Autodesk Inventor part; units mm, degrees
ref_plane "YZ Plane" through (0, 0, 0) normal (1, 0, 0) x (0, 1, 0)
ref_plane "XZ Plane" through (0, 0, 0) normal (0, 1, 0) x (-1, 0, 0)
ref_plane "XY Plane" through (0, 0, 0) normal (0, 0, 1) x (1, 0, 0)
sketch "Sketch1" plane through (0, 0, 0) normal (0, 0, 1) x (1, 0, 0)
  line L0 (0, 0) -> (71, 0)
  line L1 (71, 0) -> (71, 72.4)
  line L2 (71, 72.4) -> (0, 72.4)
  line L3 (0, 72.4) -> (0, 0)
  dimension "d0" = 71
  dimension "d1" = 72.4
extrude "Extrusion1" add sketch "Sketch1" along normal blind 10
sketch "Sketch2" plane through (0, 0, 10) normal (0, 0, 1) x (1, 0, 0)
  line L0 (71, 0) -> (71, 72.4)
  line L1 (71, 12.4) -> (81, 12.4)
  line L2 (81, 12.4) -> (81, 52.4)
  line L3 (81, 52.4) -> (71, 52.4)
  line L4 (71, 52.4) -> (71, 12.4)
  line L5 (71, 72.4) -> (0, 72.4)
  circle A0 centre (76, 32.4) radius 2.5
  line L6 (0, 0) -> (71, 0)
  point P0 (81, 32.4)
  point P1 (76, 52.4)
  dimension "d4" = 10
  dimension "d5" = 40
  dimension "d7" = 5
  dimension "d53" = 20
extrude "Extrusion2" add sketch "Sketch2" against normal blind 10
sketch "Sketch3" plane through (0, 0, 10) normal (0, 0, 1) x (1, 0, 0)
  line L0 (71, 52.4) -> (81, 52.4)
  line L1 (71, 12.4) -> (81, 12.4)
  line L2 (81, 52.4) -> (71, 52.4)
  line L3 (71, 52.4) -> (71, 12.4)
  line L4 (71, 12.4) -> (81, 12.4)
  line L5 (81, 12.4) -> (81, 52.4)
  point P0 (0, 0)
extrude "Extrusion3" cut sketch "Sketch3" against normal blind 5
sketch "Sketch10" plane through (0, 0, 0) normal (0, 0, -1) x (-1, 0, 0)
  line L0 (0, 72.4) -> (0, 0)
  line L1 (0, 12.4) -> (10, 12.4)
  line L2 (10, 12.4) -> (10, 52.4)
  line L3 (10, 52.4) -> (0, 52.4)
  line L4 (0, 52.4) -> (0, 12.4)
  circle A0 centre (5, 32.4) radius 2.5
  point P0 (-81, 12.4)
  point P1 (10, 32.4)
  point P2 (5, 12.4)
  dimension "d40" = 10
  dimension "d41" = 40
  dimension "d42" = 5
extrude "Extrusion10" add sketch "Sketch10" against normal blind 5
sketch "Sketch11" plane through (0, 0, 0) normal (0, 0, -1) x (-1, 0, 0)
  line L0 (-71, 72.4) -> (0, 72.4)
  line L1 (-15.5, 72.4) -> (-55.5, 72.4)
  line L2 (-55.5, 72.4) -> (-55.5, 82.4)
  line L3 (-55.5, 82.4) -> (-15.5, 82.4)
  line L4 (-15.5, 82.4) -> (-15.5, 72.4)
  circle A0 centre (-35.5, 77.4) radius 2.5
  point P0 (0, 0)
  point P1 (-35.5, 82.4)
  point P2 (-35.5, 72.4)
  point P3 (-15.5, 77.4)
  dimension "d46" = 40
  dimension "d47" = 10
  dimension "d48" = 5
extrude "Extrusion11" add sketch "Sketch11" against normal blind 5
sketch "Sketch12" plane through (0, 0, 0) normal (0, 0, -1) x (-1, 0, 0)
  line L0 (0, 0) -> (-71, 0)
  line L1 (-55.5, 0) -> (-15.5, 0)
  line L2 (-15.5, 0) -> (-15.5, -10)
  line L3 (-15.5, -10) -> (-55.5, -10)
  line L4 (-55.5, -10) -> (-55.5, 0)
  circle A0 centre (-35.5, -5) radius 2.5
  point P0 (-55.5, 82.4)
  point P1 (-15.5, 82.4)
  point P2 (-35.5, -10)
  point P3 (-55.5, -5)
  dimension "d54" = 10
  dimension "d55" = 5
extrude "Extrusion12" add sketch "Sketch12" against normal blind 5
properties part number "SP002" material "ABS Plastic"
Can you work these out from the model? Positions are in its coordinate system, mm. A direction names the side the tool comes from. Coordinates: 2 decimals unless noted, no trailing zeros. Loops run counter-clockwise (first coordinate to the right, second up) from the corner with the lowest first, then second, coordinate; pieces in that order, holes last. Notation, with made-up numbers: (26, 3.5) - (85, 3.5) arc R13 cw to (85, 23.5) - close; hole circle Ø11 at (23.25, -37). An arc over 180 degrees is marked (long way). Answer as CSV lines item,"result". Start each with the question number.
1) Which directions (+Z, -Z, +X, -X, +Y, -Y) give clear straight access to the entire face, cutting with the end or side of a thin tool? Please do faces 4 (the flat face through (36, 74, 5)), 5 (the flat face through (15.5, -5, 2)), 6 (the flat face through (76, 52.4, 3)), 7 (the flat face through (-8, 33, 5)).
2) Suppose I cut it at A-A (x = -5). Please give me the cut outline in (y, z).
3) Suppose I cut it at D-D (y = -5). Please give me the cut outline in (x, z), plus the area to 3 significant figures.
4) Thinking about a two-plate mould opening in Y: for faces 1 (the cylindrical face through (-6.34, 34.51, 2.46)), 2 (the flat face through (35, 37, 10)), 3 (the flat face through (35, -10, 2)), which applies, pulls with the +Y half, pulls with the -Y half, needs draft (parallel to the pull), parting line crosses it, or undercut?
5) For pin 1 (5.5 mm diameter, centred on x = 76.5, z = 1.5, fed in from -Y); pin 2 (4 mm diameter, centred on x = -7, z = 2.5, fed in from +Y); pin 3 (1.5 mm diameter, centred on y = -5, z = 2, fed in from -X); pin 4 (1 mm diameter, centred on x = 63.5, y = 70, fed in from -Z), each with a flat end and sliding along its axis, tell me the tip position at first contact or that it passes through.
6) Suppose I cut it at C-C (x = 28). Please give me the cut outline in (y, z), plus the area to 3 significant figures.
7) I need wall thicknesses on line 1 (Y direction, x = 35.5, z = 3.5); line 2 (Y direction, x = 76, z = 1.85); line 3 (Y direction, x = 2, z = 7.25). Which ranges of each line are inside material? Lowest first, please. Write a range as from..to.
8) Suppose I cut it at B-B (y = 32.4). Please give me the cut outline in (x, z).
Check result:
1,face 4,"+Z, +X, -X, +Y"
1,face 5,"+Z, -Z, -X, -Y"
1,face 6,"+Z, -Z, +X, +Y"
1,face 7,"+Z, -X, +Y, -Y"
2,outline,"(12.4, 0) - (29.9, 0) - (29.9, 5) - (12.4, 5) - close; (34.9, 0) - (52.4, 0) - (52.4, 5) - (34.9, 5) - close"
3,outline,"(15.5, 0) - (33, 0) - (33, 5) - (15.5, 5) - close; (38, 0) - (55.5, 0) - (55.5, 5) - (38, 5) - close"
3,area,"175 mm²"
4,face 1,"undercut"
4,face 2,"needs draft"
4,face 3,"pulls with the -Y half"
5,pin 1,"stops at y = 12.4"
5,pin 2,"stops at y = 52.4"
5,pin 3,"stops at x = 15.5"
5,pin 4,"stops at z = 0"
6,outline,"(-10, 0) - (82.4, 0) - (82.4, 5) - (72.4, 5) - (72.4, 10) - (0, 10) - (0, 5) - (-10, 5) - close"
6,area,"824 mm²"
7,line 1,"y = -10..-7.5, -2.5..74.9, 79.9..82.4"
7,line 2,"y = 12.4..29.9, 34.9..52.4"
7,line 3,"y = 0..72.4"
8,outline,"(-10, 0) - (-7.5, 0) - (-7.5, 5) - (-10, 5) - close; (-2.5, 0) - (73.5, 0) - (73.5, 5) - (71, 5) - (71, 10) - (0, 10) - (0, 5) - (-2.5, 5) - close; (78.5, 0) - (81, 0) - (81, 5) - (78.5, 5) - close"
